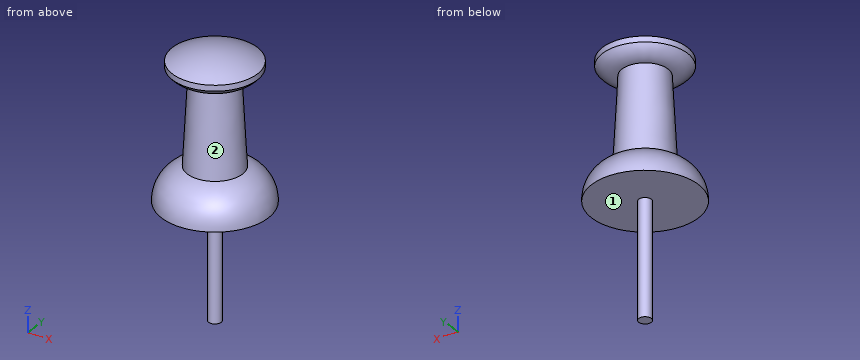
```python
from build123d import *


with BuildPart() as part:
    # Sketch2 → Revolve1 (revolve)
    with BuildSketch(Plane(origin=(0, 0, 0), x_dir=(0, 0, -1), z_dir=(1, 0, 0))):
        with BuildLine():
            Line((10, 0.55), (0, 0.55))
            Line((0, 0.55), (0, 4.65))
            ThreePointArc((0, 4.65), (-1.89487545, 4.0515006), (-3, 2.4))
            Line((-3, 2.4), (-10.5, 2))
            ThreePointArc((-10.5, 2), (-10.687950632, 2.949787938), (-11.3, 3.7))
            Line((-11.3, 3.7), (-11.8, 3.7))
            ThreePointArc((-11.8, 3.7), (-12.545594122, 1.91637679), (-12.8, 0))
            Line((-12.8, 0), (0, 0))
            Line((0, 0), (10, 0))
            Line((10, 0), (10, 0.55))
        make_face()
    revolve(axis=Axis((0, 0, -88.99), (0, 0, 1)))


solid = part.part
```
Here's how the part is built. I have some questions about the finished solid (model axes, mm). Face numbers are marked on the shaded views. Coordinates: 2 decimals unless noted, no trailing zeros. Order: outer loops, then holes, each group sorted by start corner. A loop starts at its lowest first (then second) coordinate and runs counter-clockwise, first axis right, second up. Notation, with made-up numbers: (35.5, 1.25) -> (45.5, 1.25) arc R27 cw to (45.5, 30.25) -> close; hole circle Ø2 at (11.25, 36.5). An arc over 180 degrees is marked (long way). Return JSON: item names as keys, results as strings.
1) I'm going to push flat-ended pins straight in: P1, Ø1.5, axis at x = 1, z = 1.5, coming from the +Y side; P2, Ø4, axis at x = -3.5, y = 2, coming from the +Z side; P3, Ø3, axis at x = -1.5, z = 8, coming from the -Y side. Where does each tip first touch, or does it pass through?
Conclusion:
{"P1": "stops at y = 4.51", "P2": "stops at z = 12.51", "P3": "stops at y = -2.16"}
2) If we section it at B-B on z = 10: List the corners of the cut face in (x, y) for me.
Conclusion:
{"outline": "circle Ø4.05 at (0, 0)"}
3) If we section it at A-A on z = -0.75: List the corners of the cut face in (x, y) for me, plus the area to 3 significant figures.
Conclusion:
{"outline": "circle Ø1.1 at (0, 0)", "area": "0.950 mm²"}
4) Thinking about a two-plate mould opening in Z: for the marked faces 1 and 2, which applies, +Z half, -Z half, draft (parallel to the pull), parting line (faces both ways), or undercut?
Conclusion:
{"face 1": "-Z half", "face 2": "undercut"}
5) If I drill on probe 1 along Y at (x, z) = (0, -4.5); probe 2 along Z at (x, y) = (-0.5, -2.5); probe 3 along Z at (x, y) = (-1, -2.5), over which ranges is the centre line in solid material (lowest first)?
Conclusion:
{"probe 1": "y = -0.55 to 0.55", "probe 2": "z = 0 to 2.96, 10.55 to 12.34", "probe 3": "z = 0 to 2.91, 10.59 to 12.29"}
